Study the drawing (mm; zero at the part's minimum x, y, z) and answer. Coordinates: 2 decimals unless noted, no trailing zeros. Loops run counter-clockwise (first coordinate to the right, second up) from the corner with the lowest first, then second, coordinate; pieces in that order, holes last. Notation, with made-up numbers: (63.5, 8) -> (120.5, 8) arc R19 cw to (120.5, 33) -> close; hole circle Ø4 at (6, 33). An arc over 180 degrees is marked (long way). Answer as a JSON object with one key per item and string values. Group by question number.
Q1. This flat-tipped pin is pushed along its axis until it touches: P1, Ø5, axis at x = 390, y = 12.5, coming from the -Z side. Where does it stop, or does it pass through?
Q2. The part is cut by section A-A on y = 14.75. State how many separate pieces and enclosed holes the cut face has, and give its area (3 significant figures).
Q3. Straight lines are drawn through the part: line 1 along Z through (x, y) = (221, 12); line 2 along X through (y, z) = (13.75, 343) (1 decimal); line 3 along X through (y, z) = (18.25, 80.5) (1 decimal). For each, find the intervals that lie inside material, in ascending order. Write a range as [from, to].
Q4. The part is cut by section B-B on x = 377. Write down the section's boundary in (y, z).
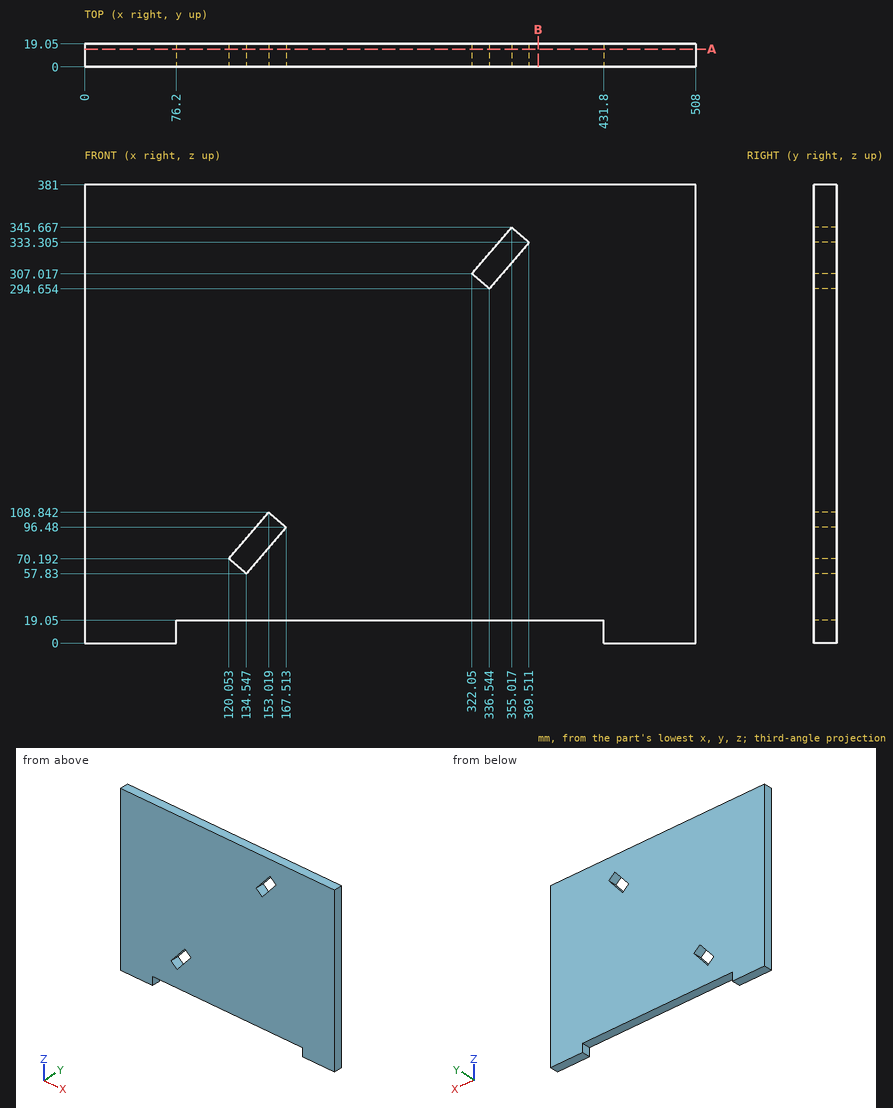
Final values:
{
 "1": {"P1": "stops at z = 19.05"},
 "2": {"separate pieces": "1", "enclosed holes": "2", "area": "185,000 mm2"},
 "3": {"line 1": "z = [19.05, 381]", "line 2": "x = [0, 352.7], [358.1, 508]", "line 3": "x = [0, 128.8], [153.9, 508]"},
 "4": {"outline": "(0, 19.05) -> (19.05, 19.05) -> (19.05, 381) -> (0, 381) -> close"}
}
